Source: CAD feature listing. Evaluate the final solid. Frame: model axes, mm. Give positions to 0.01 mm unless a question says otherwise; leave off trailing zeros. Loops run counter-clockwise (first coordinate to the right, second up) from the corner with the lowest first, then second, coordinate; pieces in that order, holes last. Notation, with made-up numbers: (-40, 72.25) -> (5, 72.25) arc R29 ccw to (5, 100.25) -> close; hole circle Ø10 at (24, -30.5). An arc over 180 degrees is marked (long way). Put each result on its own line as item: value.
```python
from build123d import *

# Parameters (mm, degrees)
SKETCH1_W           = 50
SKETCH1_H           = 50
SKETCH1_R           = 1.5
BOSS_EXTRUDE1_DEPTH = 0.7
FILLET1_R           = 10
SKETCH2_W           = 12
SKETCH2_H           = 12
SKETCH2_W_2         = 9.8
SKETCH2_H_2         = 9.8
BOSS_EXTRUDE2_DEPTH = 0.01


with BuildPart() as part:
    # Sketch1 → Boss-Extrude1 (new body)
    with BuildSketch(Plane(origin=(0, 0, 0), x_dir=(1, 0, 0), z_dir=(0, 1, 0))):
        Rectangle(SKETCH1_W, SKETCH1_H)
        with Locations(Location((-17, 17, 0), (0, 0, 270))):
            Circle(SKETCH1_R, mode=Mode.SUBTRACT)
        with Locations(Location((17, 17, 0), (0, 0, 270))):
            Circle(SKETCH1_R, mode=Mode.SUBTRACT)
        with Locations(Location((17, -17, 0), (0, 0, 270))):
            Circle(SKETCH1_R, mode=Mode.SUBTRACT)
        with Locations(Location((-17, -17, 0), (0, 0, 270))):
            Circle(SKETCH1_R, mode=Mode.SUBTRACT)
    extrude(amount=BOSS_EXTRUDE1_DEPTH)

    # Fillet1
    fillet1_edges = [part.edges().sort_by_distance(p)[0] for p in [
        (-25, 0.35, -25),
        (25, 0.35, -25),
        (25, 0.35, 25),
        (-25, 0.35, 25),
    ]]
    fillet(fillet1_edges, radius=FILLET1_R)

    # Sketch2 → Boss-Extrude2 (add)
    with BuildSketch(Plane(origin=(0, 0.7, 0), x_dir=(1, 0, 0), z_dir=(0, 1, 0))):
        Rectangle(SKETCH2_W, SKETCH2_H)
        Rectangle(SKETCH2_W_2, SKETCH2_H_2, mode=Mode.SUBTRACT)
    extrude(amount=BOSS_EXTRUDE2_DEPTH)


solid = part.part
```
(1) Draft query along Z for faces 1 (the cylindrical face through (-16.93, 0.35, -18.5)), 2 (the cylindrical face through (-22.15, 0.35, 21.99)), 3 (the flat face through (0, 0, 0)). Return one class per face: released by +Z, released by -Z, zero draft, split by the parting line, or undercut.
Calculated:
face 1: undercut
face 2: released by +Z
face 3: zero draft
(2) First-contact query: P1, Ø5, axis at x = 17, z = 17, coming from the +Y side. Flat tip, straight axial feed; report the tip coordinate or a pass-through.
Calculated:
P1: stops at y = 0.7
(3) Line query: probe 1 along X at (y, z) = (0.4, -17); probe 2 along Y at (x, z) = (-19, 17.5); probe 3 along X at (y, z) = (0.55, 17.5). Output: solid intervals per line, ascending. Write a range as from..to.
Calculated:
probe 1: x = -24.8..-18.5, -15.5..15.5, 18.5..24.8
probe 2: y = 0..0.7
probe 3: x = -24.68..-18.41, -15.59..15.59, 18.41..24.68
(4) Section B-B on x = -17. Return loops of the section in (y, z), then the cut area to 3 significant figures.
Calculated:
outline: (0, -24.8) -> (0.7, -24.8) -> (0.7, -18.5) -> (0, -18.5) -> close; (0, -15.5) -> (0.7, -15.5) -> (0.7, 15.5) -> (0, 15.5) -> close; (0, 18.5) -> (0.7, 18.5) -> (0.7, 24.8) -> (0, 24.8) -> close
area: 30.5 mm²
(5) Section A-A on y = 0.25. Return loops of the section in (x, z).
Calculated:
outline: (-25, -15) arc R10 ccw to (-15, -25) -> (15, -25) arc R10 ccw to (25, -15) -> (25, 15) arc R10 ccw to (15, 25) -> (-15, 25) arc R10 ccw to (-25, 15) -> close; hole circle Ø3 at (-17, -17); hole circle Ø3 at (-17, 17); hole circle Ø3 at (17, -17); hole circle Ø3 at (17, 17)
(6) Section C-C on z = 17. Return loops of the section in (x, y).
Calculated:
outline: (-24.8, 0) -> (-18.5, 0) -> (-18.5, 0.7) -> (-24.8, 0.7) -> close; (-15.5, 0) -> (15.5, 0) -> (15.5, 0.7) -> (-15.5, 0.7) -> close; (18.5, 0) -> (24.8, 0) -> (24.8, 0.7) -> (18.5, 0.7) -> close
